```python
from build123d import *

# Parameters (mm, degrees)
ESQUISSE1_R        = 7.5
BOSS_EXTRU_1_DEPTH = 7
ESQUISSE2_R        = 2.5
BOSS_EXTRU_2_DEPTH = 5
CONG_1_R           = 0.5


with BuildPart() as part:
    # Esquisse1 → Boss.-Extru.1 (new body)
    with BuildSketch(Plane.XY):
        Circle(ESQUISSE1_R)
    extrude(amount=BOSS_EXTRU_1_DEPTH)

    # Esquisse2 → Boss.-Extru.2 (add)
    with BuildSketch(Plane.XY.offset(7)):
        Circle(ESQUISSE2_R)
    extrude(amount=BOSS_EXTRU_2_DEPTH)

    # Congé1
    cong_1_edges = [part.edges().sort_by_distance(p)[0] for p in [
        (-7.5, 0, 7),
        (-2.5, 0, 7),
        (-2.5, 0, 12),
    ]]
    fillet(cong_1_edges, radius=CONG_1_R)


solid = part.part
```
Check sheet for the modelled part. Datum: model origin and axes. Units: mm. A direction names the side the tool comes from. Give positions to 0.01 mm unless a question says otherwise; leave off trailing zeros. Write each loop counter-clockwise with the first axis right and the second up, starting at its lowest first coordinate (ties: lowest second). Pieces come first, ordered by that corner, then holes.
Item 1: Access from +Z, -Z, +X, -X, +Y, -Y to the whole of each face (thin tool, end or side, straight path). Record for faces 1 (the face through (-7.493, 0.33, 3.204)), 2 (the face through (-0.54, -2.44, 9.47)).
Item 2: Scan lines: L1, parallel to Z at x = -0.5, y = 2; L2, parallel to Z at x = -3.25, y = 2; L3, parallel to Y at x = 0.5, z = 10.5. Record each from-to range of solid material in increasing order.
Item 3: Cross-section at C-C (z = 3.5). Enter the section's corners in (x, y), and give its area (3 significant figures).
Item 4: Cross-section at D-D (z = 8). Enter the section's corners in (x, y).
Item 5: Gauge pin test, flat ends, axial feed: pin 1 (1.5 mm diameter, centred on y = 3, z = 6.5, fed in from +X); pin 2 (5 mm diameter, centred on x = -3, z = 3, fed in from +Y); pin 3 (1.5 mm diameter, centred on y = 1.5, z = 2.5, fed in from +X). Record the tip position at first contact, or that the pin passes through.
Item 6: Cross-section at A-A (x = 0). Enter the section's corners in (y, z).
Report:
1. face 1: +Z, -Z
1. face 2: +Z
2. L1: z = 0 to 12
2. L2: z = 0 to 7
2. L3: y = -2.45 to 2.45
3. outline: circle Ø15 at (0, 0)
3. area: 177 mm2
4. outline: circle Ø5 at (0, 0)
5. pin 1: stops at x = 7.15
5. pin 2: stops at y = 7.48
5. pin 3: stops at x = 7.46
6. outline: (-7.5, 0) - (7.5, 0) - (7.5, 6.5) arc R0.5 ccw to (7, 7) - (3, 7) arc R0.5 cw to (2.5, 7.5) - (2.5, 11.5) arc R0.5 ccw to (2, 12) - (-2, 12) arc R0.5 ccw to (-2.5, 11.5) - (-2.5, 7.5) arc R0.5 cw to (-3, 7) - (-7, 7) arc R0.5 ccw to (-7.5, 6.5) - close
